Could you check a few things on this drawing? It's one solid part, dimensions in mm from its lowest x, y, z. Round coordinates to 2 decimals unless told otherwise and drop trailing zeros. Order: outer loops, then holes, each group sorted by start corner. A loop starts at its lowest first (then second) coordinate and runs counter-clockwise, first axis right, second up.
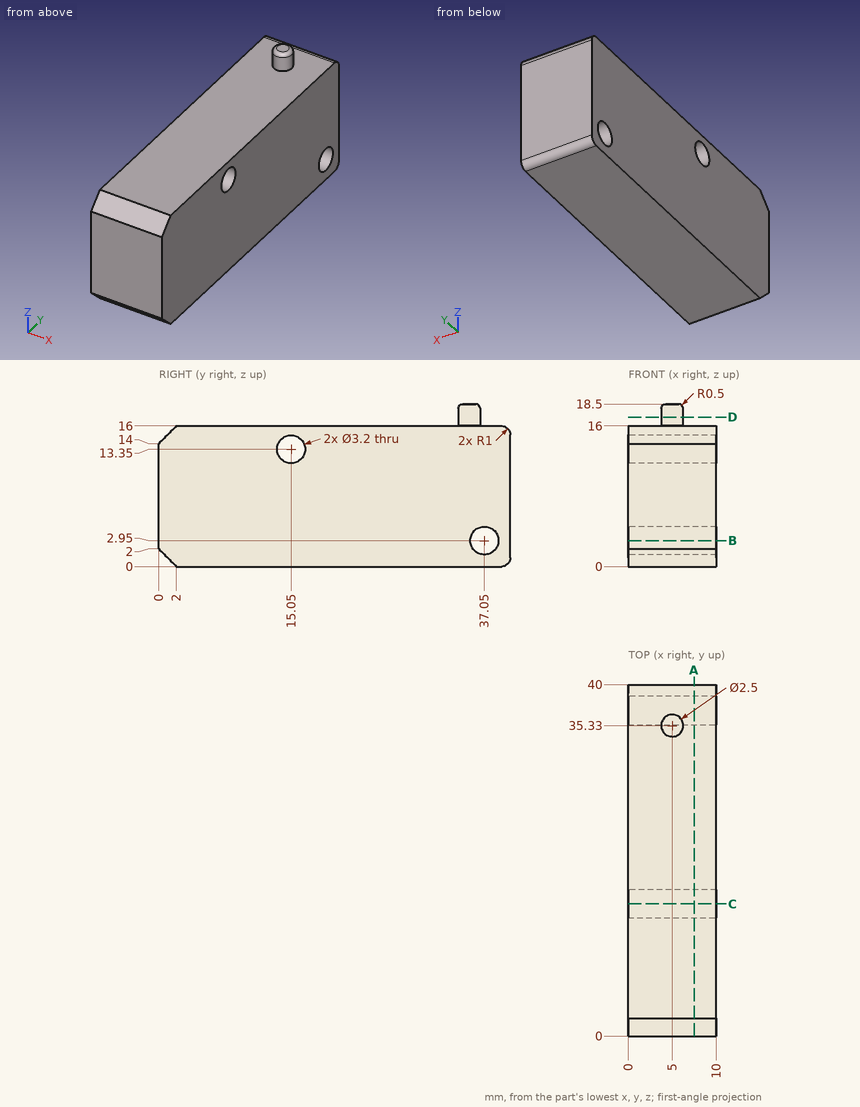
(1) I want a section at D-D, the plane z = 17. List the corners of the cut face in (x, y) for me, plus the area to 3 significant figures.
(2) I want a section at B-B, the plane z = 2.95. List the corners of the cut face in (x, y) for me, plus the area to 3 significant figures.
(3) I want a section at A-A, the plane x = 7.5. List the corners of the cut face in (y, z) for me, plus the area to 3 significant figures.
(4) I want a section at C-C, the plane y = 15.05. List the corners of the cut face in (x, z) for me, plus the area to 3 significant figures.
(5) Please list where these lines run through material, in increasing order: probe 1 along Z at (x, y) = (2.5, 37.05); probe 2 along Z at (x, y) = (4, 15.05); probe 3 along Y at (x, z) = (8.75, 13.25).
(6) I'm going to push flat-ended pins straight in: pin 1 Ø1.5 at (x, z) = (3.5, 16.5) entering from +Y; pin 2 Ø4 at (x, y) = (1, 27.5) entering from +Z. Where does each tip first touch, or does it pass through?
Ans:
1. outline: circle Ø2.5 at (5, 35.33)
1. area: 4.91 mm2
2. outline: (0, 0) - (10, 0) - (10, 35.45) - (0, 35.45) - close; (0, 38.65) - (10, 38.65) - (10, 40) - (0, 40) - close
2. area: 368 mm2
3. outline: (0, 2) - (2, 0) - (39, 0) arc R1 ccw to (40, 1) - (40, 15) arc R1 ccw to (39, 16) - (2, 16) - (0, 14) - close; hole circle Ø3.2 at (15.05, 13.35); hole circle Ø3.2 at (37.05, 2.95)
3. area: 619 mm2
4. outline: (0, 0) - (10, 0) - (10, 11.75) - (0, 11.75) - close; (0, 14.95) - (10, 14.95) - (10, 16) - (0, 16) - close
4. area: 128 mm2
5. probe 1: z = 0 to 1.35, 4.55 to 16
5. probe 2: z = 0 to 11.75, 14.95 to 16
5. probe 3: y = 0 to 13.45, 16.65 to 40
6. pin 1: stops at y = 39.66
6. pin 2: stops at z = 16
